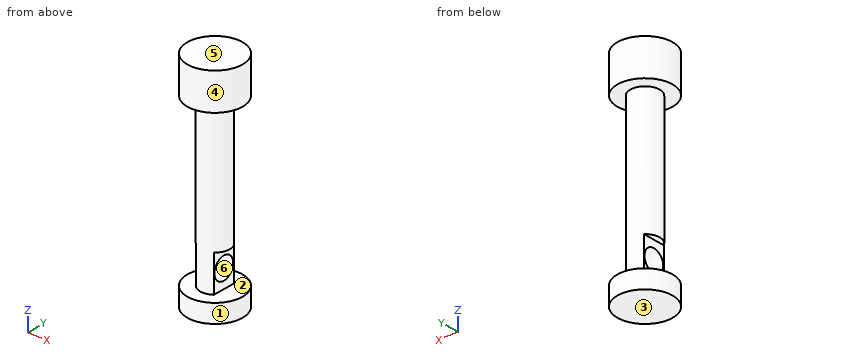
from build123d import *

# Parameters (mm, degrees)
CORTE_EXTRUS_O1_DEPTH      = 64.639610307
CORTE_EXTRUS_O1_DEPTH_BACK = 64.639610307
ESBO_O2_R                  = 6
CORTE_EXTRUS_O2_START      = -30
CORTE_EXTRUS_O2_DEPTH      = 30
BOSS_EXTRUDE1_START        = -10
SKETCH1_R                  = 15
BOSS_EXTRUDE1_DEPTH        = 10


with BuildPart() as part:
    # Esboço1 → Revolução1 (revolve)
    with BuildSketch(Plane(origin=(0, 0, 0), x_dir=(0, 0, -1), z_dir=(1, 0, 0)), mode=Mode.PRIVATE) as revolu_o1_sk:
        Polygon((-60, 0), (60, 0), (60, 8), (-40, 8), (-40, 15), (-60, 15), align=None)
    revolve(revolu_o1_sk.sketch.rotate(Axis((0, 0, 60), (0, 0, -1)), 90), axis=Axis((0, 0, 60), (0, 0, -1)))

    # Esboço2 → Corte-extrusão1 (cut, two sides: drawn at the far end of the back side and taken through both)
    with BuildSketch(Plane(origin=(0, 0, 0), x_dir=(0, 0, -1), z_dir=(1, 0, 0)).offset(-CORTE_EXTRUS_O1_DEPTH_BACK)):
        with Locations((40, 0)):
            Circle(ESBO_O2_R)
    extrude(amount=CORTE_EXTRUS_O1_DEPTH + CORTE_EXTRUS_O1_DEPTH_BACK, mode=Mode.SUBTRACT)

    # Esboço3 → Corte-extrusão2 (cut)
    with BuildSketch(Plane(origin=(0, 0, -60), x_dir=(-1, 0, 0), z_dir=(0, 0, -1)).offset(CORTE_EXTRUS_O2_START)):
        with BuildLine():
            Line((-4.839112888, -6.370477726), (-4.839112888, 6.370477726))
            ThreePointArc((-4.839112888, 6.370477726), (-8, 0), (-4.839112888, -6.370477726))
        make_face()
        with BuildLine():
            ThreePointArc((8, 0), (7.166341574, 3.555776771), (4.839112888, 6.370477726))
            Line((4.839112888, 6.370477726), (4.839112888, -6.370477726))
            ThreePointArc((4.839112888, -6.370477726), (7.166341574, -3.555776771), (8, 0))
        make_face()
    extrude(amount=CORTE_EXTRUS_O2_DEPTH, mode=Mode.SUBTRACT)

    # Sketch1 → Boss-Extrude1 (add)
    with BuildSketch(Plane(origin=(0, 0, -60), x_dir=(-1, 0, 0), z_dir=(0, 0, -1)).offset(BOSS_EXTRUDE1_START)):
        with Locations(Location((0, 0, 0), (0, 0, 180))):
            Circle(SKETCH1_R)
    extrude(amount=BOSS_EXTRUDE1_DEPTH)


solid = part.part
Build history of the part. All positions in model axes, mm. Face numbers are marked on the shaded views. A direction names the side the tool comes from. Coordinates: 2 decimals unless noted, no trailing zeros. Write each loop counter-clockwise with the first axis right and the second up, starting at its lowest first coordinate (ties: lowest second). Pieces come first, ordered by that corner, then holes.
(1) Drill centre lines: line 1 (Z direction, x = 2.75, y = 0); line 2 (Z direction, x = -9.25, y = -8); line 3 (Y direction, x = -0.25, z = -40). Where is each one in solid material? Low to high.
(2) Pin check, flat tips, straight feed: pin 1 Ø8 at (y, z) = (-2, 27.5) entering from -X; pin 2 Ø9.5 at (y, z) = (0, -40) entering from +X; pin 3 Ø10 at (y, z) = (-1.5, -35.5) entering from +X; pin 4 Ø2 at (y, z) = (1, 9) entering from +X. Stop position of each tip, or through.
(3) Cut at A-A on y = 0. List the corners of the cut face in (x, z), and give its area (3 significant figures).
(4) Mould opens along Z. For the marked faces 3, 4, 5 and 6 say: pulls with the +Z half, pulls with the -Z half, needs draft (parallel to the pull), parting line crosses it, or undercut.
(5) Cut at D-D on y = -10.5. List the corners of the cut face in (x, z).
(6) Cut at C-C on x = 0. List the corners of the cut face in (y, z), and give its area (3 significant figures).
(7) 3-axis set-ups, long thin cutter, end or side, ignore diameter. For the marked faces 1 and 2: which of +Z, -Z, +X, -X, +Y, -Y reach the whole face in a straight line?
(8) Cut at B-B on z = -40. List the corners of the cut face in (x, y), and give its area (3 significant figures).
Working result:
1. line 1: z = -60 to -46, -34 to 60
1. line 2: z = -60 to -50, 40 to 60
1. line 3: y = -8 to -6, 6 to 8
2. pin 1: stops at x = -8
2. pin 2: passes through
2. pin 3: stops at x = 4.84
2. pin 4: stops at x = 8
3. outline: (-15, -60) - (15, -60) - (15, -50) - (4.84, -50) - (4.84, -46) - (-4.84, -46) - (-4.84, -50) - (-15, -50) - close; (-15, 40) - (-8, 40) - (-8, -30) - (-4.84, -30) - (-4.84, -34) - (4.84, -34) - (4.84, -30) - (8, -30) - (8, 40) - (15, 40) - (15, 60) - (-15, 60) - close
3. area: 2,100 mm2
4. face 3: pulls with the -Z half
4. face 4: needs draft
4. face 5: pulls with the +Z half
4. face 6: undercut
5. outline: (-10.71, -60) - (10.71, -60) - (10.71, -50) - (-10.71, -50) - close; (-10.71, 40) - (10.71, 40) - (10.71, 60) - (-10.71, 60) - close
6. outline: (-15, -60) - (15, -60) - (15, -50) - (8, -50) - (8, 40) - (15, 40) - (15, 60) - (-15, 60) - (-15, 40) - (-8, 40) - (-8, -50) - (-15, -50) - close; hole circle Ø12 at (0, -40)
6. area: 2,230 mm2
7. face 1: +Z, -Z
7. face 2: none
8. outline: (-4.84, -6.37) arc R8 ccw to (4.84, -6.37) - (4.84, -6) - (-4.84, -6) - close; (-4.84, 6) - (4.84, 6) - (4.84, 6.37) arc R8 ccw to (-4.84, 6.37) - close
8. area: 28.7 mm2
